CAD build for the part. Positions are in the model's coordinates, mm. A direction names the side the tool comes from. Coordinates: 2 decimals unless noted, no trailing zeros. Loops run counter-clockwise (first coordinate to the right, second up) from the corner with the lowest first, then second, coordinate; pieces in that order, holes last. Notation, with made-up numbers: (-18.5, 64) -> (20.5, 64) arc R33 cw to (20.5, 98) -> close; hole circle Ø1 at (6, 19.5). An arc over 180 degrees is marked (long way). Write item = value, one per line. Start each with the question number.
(1) Band-saw the part on B-B (z = 285). Write the cut outline in (x, y).
(2) Pull direction X, two halves, no side cores. Call faces 1 (the face through (0, 24, 450)), 2 (the face through (25, 0, 235)), 3 (the face through (0, 23, 235)): +X half, -X half, draft (parallel to the pull), parting line (faces both ways), or undercut.
(3) Tool access for faces 4 (the face through (0, -23, 235)), 5 (the face through (-25, 0, 235)): list every direction of +Z, -Z, +X, -X, +Y, -Y with a clear straight run to the whole face (end or side of a thin tool).
(4) Drill centre lines: line 1 (Z direction, x = 16, y = -24.2); line 2 (Y direction, x = -9, z = 193.5). Where is each one in solid material? Low to high. Write a range as from..to.
(5) Flat gauge pin, fed straight in: P1, Ø3, axis at x = -16, z = 93, coming from the +Y side. Where does the tip first touch, or does it go through?
(6) Band-saw the part on A-A (y = -17.5). Write the cut outline in (x, z), and give its area (3 significant figures).
Autodesk Inventor part; units mm, degrees
ref_plane "Start Plane" through (0, 0, 25) normal (0, 0, 1) x (1, 0, 0)
ref_plane "End Plane" through (0, 0, 450) normal (0, 0, 1) x (1, 0, 0)
ref_plane "Work Plane4" through (0, 20, 25) normal (0, 0, -1) x (-1, 0, 0)
ref_plane "Start Plane" through (0, 0, 25) normal (0, 0, 1) x (1, 0, 0)
ref_plane "End Plane" through (0, 0, 450) normal (0, 0, 1) x (1, 0, 0)
sketch "Sketch" plane through (0, 0, 0) normal (0, 0, 1) x (1, 0, 0)
  line L0 (-25, -21) -> (-25, 21)
  line L1 (-21, 25) -> (21, 25)
  line L2 (25, 21) -> (25, -21)
  line L3 (21, -25) -> (-21, -25)
  arc A0 (-25, -21) -> (-21, -25) centre (-21, -21) ccw
  arc A1 (25, 21) -> (21, 25) centre (21, 21) ccw
  arc A2 (-21, 25) -> (-25, 21) centre (-21, 21) ccw
  arc A3 (21, -25) -> (25, -21) centre (21, -21) ccw
  arc A4 (-21, 23) -> (-23, 21) centre (-21, 21) ccw
  line L4 (-21, 23) -> (21, 23)
  arc A5 (23, 21) -> (21, 23) centre (21, 21) ccw
  line L5 (23, 21) -> (23, -21)
  arc A6 (21, -23) -> (23, -21) centre (21, -21) ccw
  line L6 (21, -23) -> (-21, -23)
  arc A7 (-23, -21) -> (-21, -23) centre (-21, -21) ccw
  line L7 (-23, -21) -> (-23, 21)
  line L8 (0, 36.1598) -> (0, -36.1598) construction
  line L9 (-36.1598, 0) -> (36.1598, 0) construction
  dimension "d7" = 4
  dimension "d9" = 50
  dimension "d11" = 50
  dimension "d12" = 2
  dimension "d15" = 25
  dimension "d16" = 25
extrude "Body" add sketch "Sketch" along normal up to surface (425 mm away) from surface at 25
sketch "Sketch3" plane through (0, 0, 0) normal (0, 0, 1) x (1, 0, 0)
  line L0 (0, 0) -> (10, 0)
ref_plane "Work Plane3" through (0, 0, 0) normal (0, -1, 0) x (1, 0, 0)
sketch "Sketch4" plane through (0, 0, 0) normal (0, -1, 0) x (1, 0, 0)
  line L0 (-2, 25) -> (12, 25)
  line L1 (-2, 450) -> (12, 450)
  dimension "d18" = 425
ref_plane "Work Plane4" through (0, 20, 25) normal (0, 0, -1) x (-1, 0, 0)
split "Split1" plane through (0, 20, 25) removes the side toward (0, 0, -1)
sketch "Sketch5" plane through (21, 25, 450) normal (0, 1, 0) x (1, 0, 0)
  line L0 (-5, 357) -> (-37, 357)
  line L1 (-37, 357) -> (-37, 393)
  line L2 (-37, 393) -> (-5, 393)
  line L3 (-5, 393) -> (-5, 357)
  line L4 (-42, 0) -> (0, 0)
  line L5 (0, 425) -> (0, 0)
  line L6 (-42, 425) -> (0, 425)
  line L7 (-42, 425) -> (-42, 0)
  line L8 (0, 425) -> (-42, 425)
  line L9 (-21, 425) -> (-21, 412.7282)
  point P0 (-21, 450)
  dimension "d19" = 32
  dimension "d20" = 32
  dimension "d21" = 36
hole "Hole1" at (16, 25, 93) at (16, 25, 57) at (-16, 25, 57) at (-16, 25, 93) direction (0, -1, 0) diameter 5 depth 50
equation "\"d7\" = G_IR"
equation "\"d9\" = G_W"
equation "\"d11\" = G_H"
equation "\"d12\" = G_T"
equation "\"d15\" = 0.5 * d9"
equation "\"d16\" = 0.5 * d11"
equation "\"d3\" = G_L"
equation "\"G_W\" = 50"
equation "\"G_H\" = 50"
equation "\"G_T\" = 2"
equation "\"G_IR\" = 4"
equation "\"G_L\" = d18"
equation "\"G_OFFSET_START\" = -25"
equation "\"G_OFFSET_END\" = 0"
equation "\"d13\" = -G_OFFSET_START"
properties part number "ISO 10799-2 - 50x50x2 - 425" material "Steel, Galvanized"
Findings below:
q1.outline = (-25, -21) arc R4 ccw to (-21, -25) -> (21, -25) arc R4 ccw to (25, -21) -> (25, 21) arc R4 ccw to (21, 25) -> (-21, 25) arc R4 ccw to (-25, 21) -> close; hole (-23, -21) arc R2 ccw to (-21, -23) -> (21, -23) arc R2 ccw to (23, -21) -> (23, 21) arc R2 ccw to (21, 23) -> (-21, 23) arc R2 ccw to (-23, 21) -> close
q2.face_1 = draft
q2.face_2 = +X half
q2.face_3 = undercut
q3.face_4 = +Z, -Z
q3.face_5 = +Z, -Z, -X, +Y, -Y
q4.line_1 = 25..54.5, 59.5..90.5, 95.5..450
q4.line_2 = -25..-23, 23..25
q5.P1 = through
q6.outline = (-25, 25) -> (-23, 25) -> (-23, 450) -> (-25, 450) -> close; (23, 25) -> (25, 25) -> (25, 450) -> (23, 450) -> close
q6.area = 1,700 mm²
